Geometry: final body of the model. Coordinates: model frame, mm. A direction names the side the tool comes from. Coordinates: 2 decimals unless noted, no trailing zeros. Order: outer loops, then holes, each group sorted by start corner. A loop starts at its lowest first (then second) coordinate and runs counter-clockwise, first axis right, second up. Notation, with made-up numbers: (-16, 88) - (-8, 88) arc R13 ccw to (-8, 104) - close; hole circle Ø3 at (-12, 48.25). An arc over 180 degrees is marked (long way). Use a Markdown table: item, result. Add a question column.
```python
from build123d import *

# Parameters (mm, degrees)
SKETCH_1_R                = 1.7
SKETCH_1_R_2              = 2.45
SKETCH_1_R_3              = 1.786756839
SKETCH_1_W                = 41.55
SKETCH_1_H                = 20.05
F_02_PAN_SERVO_DECK_DEPTH = 6


with BuildPart() as part:
    # Эскиз1 → 02_Pan_servo_deck (new body)
    with BuildSketch(Plane.XY):
        Polygon((-40.5, -40), (40.5, -40), (52.5, -28), (52.5, 28), (40.5, 40), (-40.5, 40), (-52.5, 28), (-52.5, -28), align=None)
        with Locations((-14.25, -5)):
            Circle(SKETCH_1_R, mode=Mode.SUBTRACT)
        with Locations((-14.25, 5)):
            Circle(SKETCH_1_R, mode=Mode.SUBTRACT)
        with Locations((35.25, -5)):
            Circle(SKETCH_1_R, mode=Mode.SUBTRACT)
        with Locations((35.25, 5)):
            Circle(SKETCH_1_R, mode=Mode.SUBTRACT)
        with Locations((-36, -25)):
            Circle(SKETCH_1_R, mode=Mode.SUBTRACT)
        with Locations((-36, 25)):
            Circle(SKETCH_1_R, mode=Mode.SUBTRACT)
        with Locations((35.25, -25)):
            Circle(SKETCH_1_R_2, mode=Mode.SUBTRACT)
        with Locations((35.25, 25)):
            Circle(SKETCH_1_R_2, mode=Mode.SUBTRACT)
        with Locations((0, 27.45)):
            Circle(SKETCH_1_R_3, mode=Mode.SUBTRACT)
        with Locations((0, -28)):
            Circle(SKETCH_1_R, mode=Mode.SUBTRACT)
        with Locations((-29, 0)):
            Circle(SKETCH_1_R, mode=Mode.SUBTRACT)
        with Locations((10.375, 0.125)):
            Rectangle(SKETCH_1_W, SKETCH_1_H, mode=Mode.SUBTRACT)
    extrude(amount=F_02_PAN_SERVO_DECK_DEPTH)


solid = part.part
```
1) Section query B-B (y = -5). Return the cut outline in (x, z), and give its area (3 significant figures).
2) First-contact query: pin 1 (2 mm diameter, centred on x = 35.25, y = -5, fed in from +Z). Flat tip, straight axial feed; report the tip coordinate or a pass-through.
3) Section query C-C (x = -29). Return the cut outline in (y, z), and give its area (3 significant figures).
4) Section query A-A (x = -14.25). Return the cut outline in (y, z), and give its area (3 significant figures).
5) Line query: line 1 (Y direction, x = 35.25, z = 1.85); line 2 (X direction, y = -2, z = 1.4); line 3 (X direction, y = -0.5, z = 3.35). Output: solid intervals per line, ascending. Write a range as from..to.
6) Draft query along Y for faces 3 (the flat face through (52.5, 0, 3)), 4 (the cylindrical face through (-13.47, 3.49, 2.96)), 5 (the flat face through (-46.6, -33.9, 3)). Return one class per face: released by +Y, released by -Y, zero draft, split by the parting line, or undercut.
7) Section query D-D (y = -25). Return the cut outline in (x, z).
8) Access query for faces 1 (the flat face through (10, 10.15, 3)), 2 (the flat face through (-12, 1, 6)). Directions: +Z, -Z, +X, -X, +Y, -Y. A direction counts if a zero-diameter tool reaches every point of the face in a straight line with its end or side. Return the directions, or none.
From the geometry:
| question | item | result |
|---|---|---|
| 1 | outline | (-52.5, 0) - (-15.95, 0) - (-15.95, 6) - (-52.5, 6) - close; (-12.55, 0) - (-10.4, 0) - (-10.4, 6) - (-12.55, 6) - close; (31.15, 0) - (33.55, 0) - (33.55, 6) - (31.15, 6) - close; (36.95, 0) - (52.5, 0) - (52.5, 6) - (36.95, 6) - close |
| 1 | area | 340 mm^2 |
| 2 | pin 1 | passes through |
| 3 | outline | (-40, 0) - (-1.7, 0) - (-1.7, 6) - (-40, 6) - close; (1.7, 0) - (40, 0) - (40, 6) - (1.7, 6) - close |
| 3 | area | 460 mm^2 |
| 4 | outline | (-40, 0) - (-6.7, 0) - (-6.7, 6) - (-40, 6) - close; (-3.3, 0) - (3.3, 0) - (3.3, 6) - (-3.3, 6) - close; (6.7, 0) - (40, 0) - (40, 6) - (6.7, 6) - close |
| 4 | area | 439 mm^2 |
| 5 | line 1 | y = -40..-27.45, -22.55..-6.7, -3.3..3.3, 6.7..22.55, 27.45..40 |
| 5 | line 2 | x = -52.5..-10.4, 31.15..52.5 |
| 5 | line 3 | x = -52.5..-30.62, -27.38..-10.4, 31.15..52.5 |
| 6 | face 3 | zero draft |
| 6 | face 4 | undercut |
| 6 | face 5 | released by -Y |
| 7 | outline | (-52.5, 0) - (-37.7, 0) - (-37.7, 6) - (-52.5, 6) - close; (-34.3, 0) - (32.8, 0) - (32.8, 6) - (-34.3, 6) - close; (37.7, 0) - (52.5, 0) - (52.5, 6) - (37.7, 6) - close |
| 8 | face 1 | +Z, -Z |
| 8 | face 2 | +Z, +X, -X, +Y, -Y |
